Could you check a few things on this drawing? It's one solid part, dimensions in mm from its lowest x, y, z. Round coordinates to 2 decimals unless told otherwise and drop trailing zeros. Loops run counter-clockwise (first coordinate to the right, second up) from the corner with the lowest first, then second, coordinate; pieces in that order, holes last.
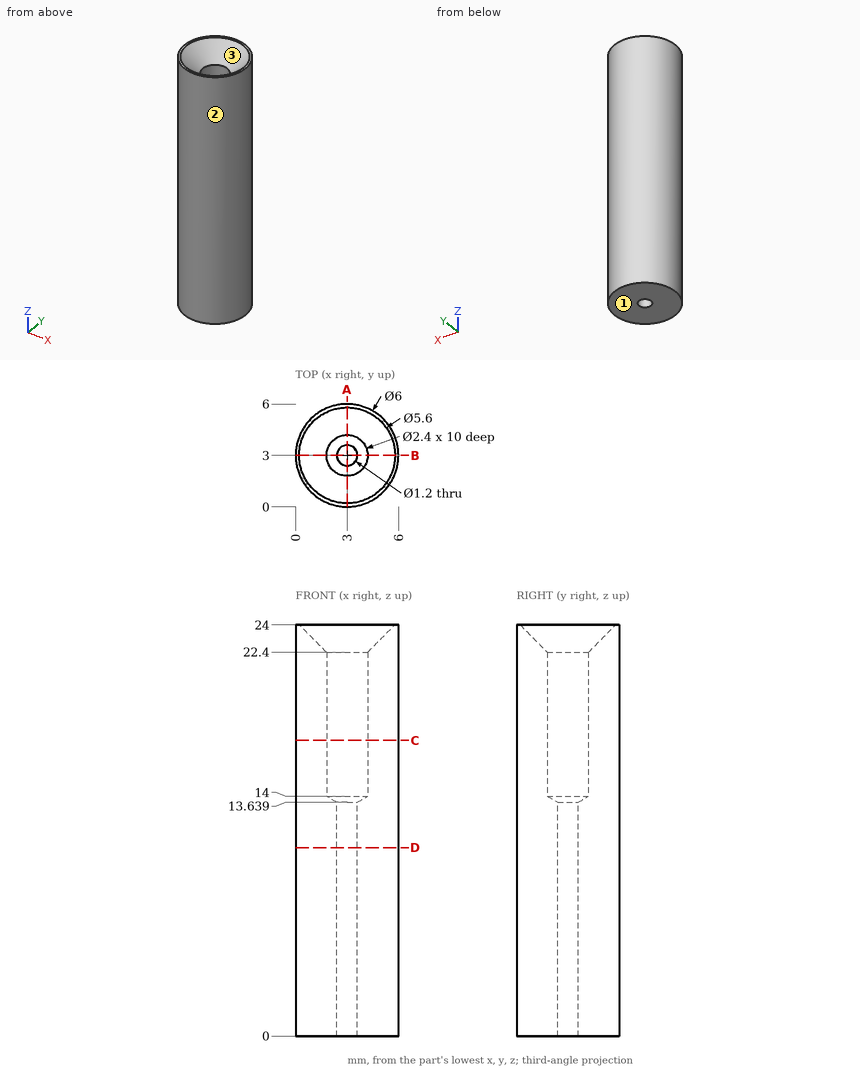
(1) Suppose I cut it at A-A (x = 3). Write out the boundary of the cut face in (y, z).
(2) For pin 1 (1.5 mm diameter, centred on y = 1, z = 5, fed in from +X); pin 2 (1 mm diameter, centred on x = 3, y = 3, fed in from -Z); pin 3 (1 mm diameter, centred on x = 5, y = 3.5, fed in from +Z), each with a flat end and sliding along its axis, tell me the tip position at first contact or that it passes through.
(3) Suppose I cut it at C-C (z = 17.25). Write out the boundary of the cut face in (x, y).
(4) Suppose I cut it at D-D (z = 11). Write out the boundary of the cut face in (x, y).
(5) We'd pull the mould along X, two halves only. Please class the marked faces 1, 2 and 3: released by +X, released by -X, zero draft, split by the parting line, or undercut.
(6) If I drill on line 1 (Y direction, x = 3, z = 19.75); line 2 (X direction, y = 2.95, z = 4.75), over which ranges is the centre line in solid material (lowest first)?
Check result:
1. outline: (0, 0) - (2.4, 0) - (2.4, 13.64) - (1.8, 14) - (1.8, 22.4) - (0.2, 24) - (0, 24) - close; (3.6, 0) - (6, 0) - (6, 24) - (5.8, 24) - (4.2, 22.4) - (4.2, 14) - (3.6, 13.64) - close
2. pin 1: stops at x = 5.73
2. pin 2: passes through
2. pin 3: stops at z = 23.76
3. outline: circle Ø6 at (3, 3); hole circle Ø2.4 at (3, 3)
4. outline: circle Ø6 at (3, 3); hole circle Ø1.2 at (3, 3)
5. face 1: zero draft
5. face 2: split by the parting line
5. face 3: undercut
6. line 1: y = 0 to 1.8, 4.2 to 6
6. line 2: x = 0 to 2.4, 3.6 to 6
